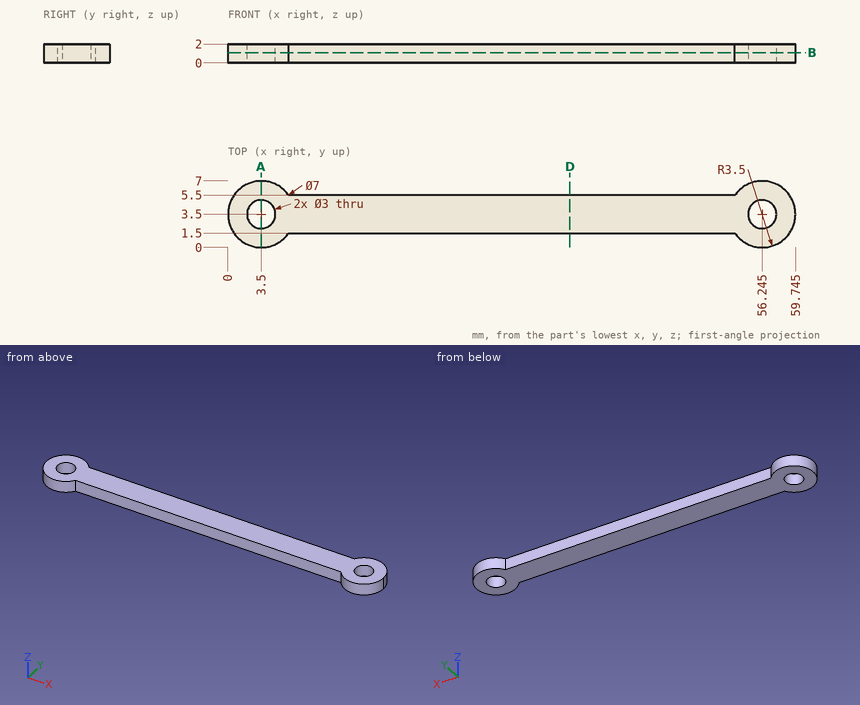
Part print with two shaded views. Sizes in mm from the minimum x, y, z corner. Coordinates: 2 decimals unless noted, no trailing zeros. Order: outer loops, then holes, each group sorted by start corner. A loop starts at its lowest first (then second) coordinate and runs counter-clockwise, first axis right, second up. Notation, with made-up numbers: M 9,-6.5 L 62,-6.5 A13 cw 62,8.5 Z; hole C -31,-28.5 d4. An arc over 180 degrees is marked long. One line per question, with ' | ' between items. Start each with the question number.
1. Cut at A-A (x = 3.5). Write the cut outline in (y, z).
2. Cut at B-B (z = 1.1). Write the cut outline in (x, y) (1 decimal).
3. Flat gauge pins, fed straight in: P1, Ø1.8, axis at x = 3.5, y = 3.5, coming from the -Z side; P2, Ø1, axis at x = 33, z = 0.5, coming from the -Y side; P3, Ø0.6, axis at x = 27.5, z = 0.5, coming from the +Y side. Where does each tip first touch, or does it go through?
4. Wall check: line 1 along X through (y, z) = (3.75, 1.5) (1 decimal); line 2 along X through (y, z) = (2.5, 0.25) (1 decimal); line 3 along Y through (x, z) = (3.5, 1.2). Give the ranges that are in metal, low to high. Write a range as [from, to].
5. Cut at D-D (x = 36). Write the cut outline in (y, z).
The answers:
1) outline: M 0,0 L 2,0 L 2,2 L 0,2 Z; M 5,0 L 7,0 L 7,2 L 5,2 Z
2) outline: M 6.4,1.5 L 53.4,1.5 A3.5 ccw long 53.4,5.5 L 6.4,5.5 A3.5 ccw long Z; hole C 3.5,3.5 d3; hole C 56.2,3.5 d3
3) P1: passes through | P2: stops at y = 1.5 | P3: stops at y = 5.5
4) line 1: x = [0, 2], [5, 54.8], [57.7, 59.7] | line 2: x = [0.1, 2.4], [4.6, 55.1], [57.4, 59.6] | line 3: y = [0, 2], [5, 7]
5) outline: M 1.5,0 L 5.5,0 L 5.5,2 L 1.5,2 Z
